```python
from build123d import *

# Parameters (mm, degrees)
SKETCH2_R                = 3.175
CUT_EXTRUDE1_DEPTH       = 6.715
CUT_EXTRUDE1_DEPTH_BACK  = 6.715
SKETCH3_R                = 6.35
SKETCH3_R_2              = 3.175
BOSS_EXTRUDE1_DEPTH      = 4.7625
BOSS_EXTRUDE1_DEPTH_BACK = 4.7625
SKETCH4_W                = 5.08
SKETCH4_H                = 5.08
BOSS_EXTRUDE2_DEPTH      = 25.4


with BuildPart() as part:
    # Sketch1 → Revolve1 (revolve)
    with BuildSketch(Plane.XY):
        with BuildLine():
            Line((0, 5.715), (0, -5.715))
            ThreePointArc((0, -5.715), (5.715, 0), (0, 5.715))
        make_face()
    revolve(axis=Axis((0, 5.715, 0), (0, -1, 0)))

    # Sketch2 → Cut-Extrude1 (cut, two sides)
    with BuildSketch(Plane(origin=(0, 0, 0), x_dir=(1, 0, 0), z_dir=(0, 1, 0))) as cut_extrude1_sk:
        Circle(SKETCH2_R)
    extrude(amount=CUT_EXTRUDE1_DEPTH, mode=Mode.SUBTRACT)
    extrude(cut_extrude1_sk.sketch, amount=-CUT_EXTRUDE1_DEPTH_BACK, mode=Mode.SUBTRACT)

    # Sketch3 → Boss-Extrude1 (add, two sides)
    with BuildSketch(Plane(origin=(0, 0, 0), x_dir=(1, 0, 0), z_dir=(0, 1, 0))) as boss_extrude1_sk:
        Circle(SKETCH3_R)
        Circle(SKETCH3_R_2, mode=Mode.SUBTRACT)
    extrude(amount=BOSS_EXTRUDE1_DEPTH)
    extrude(boss_extrude1_sk.sketch, amount=-BOSS_EXTRUDE1_DEPTH_BACK)

    # Sketch4 → Boss-Extrude2 (add)
    with BuildSketch(Plane(origin=(0, 0, 0), x_dir=(0, 0, -1), z_dir=(1, 0, 0))):
        Rectangle(SKETCH4_W, SKETCH4_H)
    extrude(amount=BOSS_EXTRUDE2_DEPTH)


solid = part.part
```
Input: part model. Units: mm. Frame: model coordinates. A direction names the side the tool comes from. Give positions to 0.01 mm unless a question says otherwise; leave off trailing zeros. Order: outer loops, then holes, each group sorted by start corner. A loop starts at its lowest first (then second) coordinate and runs counter-clockwise, first axis right, second up. Notation, with made-up numbers: (82, -11.75) - (99, -11.75) arc R22 ccw to (99, 19.25) - close; hole circle Ø3 at (-4, 81.25). An arc over 180 degrees is marked (long way). Put each result on its own line as item: value.
Item 1: Ray query, L1, parallel to Z at x = 0, y = -2.7 (3 decimals); L2, parallel to X at y = 1.1, z = 0 (3 decimals). Return the intervals inside material, ascending. Write a range as from..to.
Found:
L1: z = -6.35..-3.175, 3.175..6.35
L2: x = -6.35..-3.175, 0..25.4
Item 2: Contact query for flat-ended pins moving along their axis: pin 1 (6 mm diameter, centred on x = 21.5, z = -1.5, fed in from +Y); pin 2 (3 mm diameter, centred on y = 1, z = 3.5, fed in from -X); pin 3 (1 mm diameter, centred on x = 15.5, y = -2, fed in from +Z). Output: stop coordinate, or through.
Found:
pin 1: stops at y = 2.54
pin 2: stops at x = -6.03
pin 3: stops at z = 2.54
Item 3: Section query B-B, the plane y = -1.75. Return loops of the section in (x, z) (3 decimals), then the cut area to 3 significant figures.
Found:
outline: (5.82, -2.54) - (25.4, -2.54) - (25.4, 2.54) - (5.82, 2.54) arc R6.35 ccw (long way) to start; hole (0, -2.54) - (0, 2.54) - (1.905, 2.54) arc R3.175 ccw (long way) to (1.905, -2.54) - close
area: 207 mm^2
Item 4: Draft query along Z for faces 1 (the cylindrical face through (-6.344, 0.067, -0.279)), 2 (the flat face through (25.4, 0, 0)), 3 (the flat face through (1, 0, -2.54)). Return one class per face: +Z half, -Z half, draft (parallel to the pull), parting line (faces both ways), or undercut.
Found:
face 1: parting line
face 2: draft
face 3: undercut
Item 5: Section query D-D, the plane x = 7. Return loops of the section in (y, z).
Found:
outline: (-2.54, -2.54) - (2.54, -2.54) - (2.54, 2.54) - (-2.54, 2.54) - close
Item 6: Access query for faces 4 (the flat face through (2, 2.54, 0)), 5 (the flat face through (15, 0, 2.54)), 6 (the flat face through (2, -2.54, 0)), 7 (the flat face through (15, 0, -2.54)). Directions: +Z, -Z, +X, -X, +Y, -Y. A direction counts if a zero-diameter tool reaches every point of the face in a straight line with its end or side. Return the directions, or none.
Found:
face 4: +Y
face 5: +Z, +X, +Y, -Y
face 6: -Y
face 7: -Z, +X, +Y, -Y
Item 7: Section query C-C, the plane x = -2. Return loops of the section in (y, z), then the cut area to 3 significant figures.
Found:
outline: (-4.76, -6.03) - (4.76, -6.03) - (4.76, -2.47) - (-4.76, -2.47) - close; (-4.76, 2.47) - (4.76, 2.47) - (4.76, 6.03) - (-4.76, 6.03) - close
area: 67.8 mm^2
